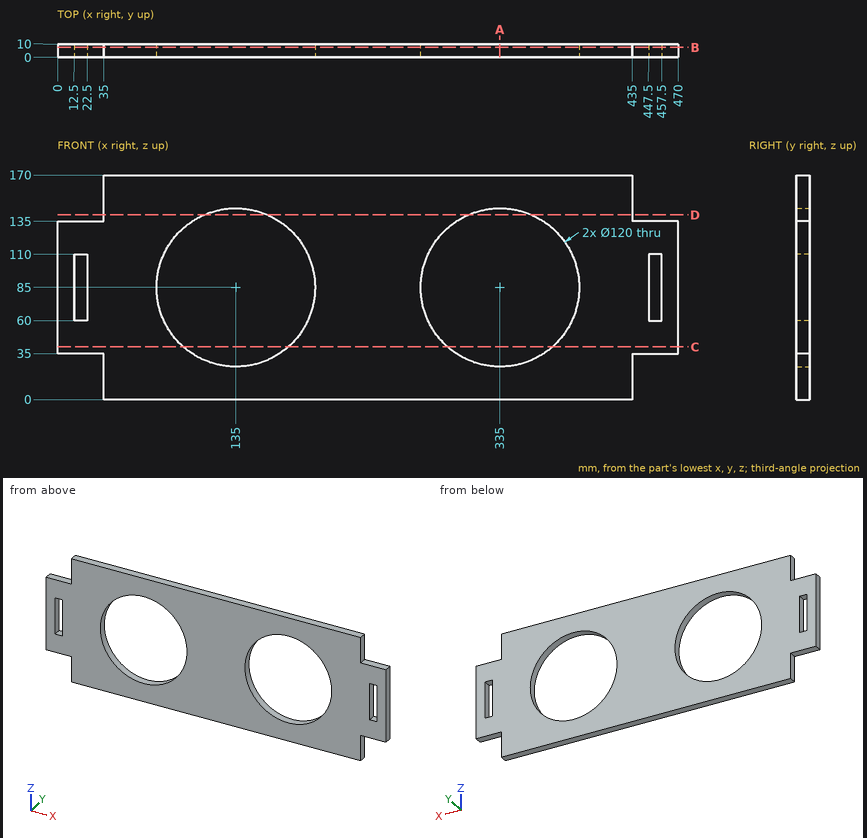
Verification items for this drawing (mm, ordinates from the low corner). Give positions to 0.01 mm unless a question says otherwise; leave off trailing zeros. Order: outer loops, then holes, each group sorted by start corner. A loop starts at its lowest first (then second) coordinate and runs counter-clockwise, first axis right, second up.
1) Cross-section at D-D (z = 140). Record the boundary of the cut face in (x, y), then the cut area to 3 significant figures.
Results are:
outline: (35, 0) - (111.02, 0) - (111.02, 10) - (35, 10) - close; (158.98, 0) - (311.02, 0) - (311.02, 10) - (158.98, 10) - close; (358.98, 0) - (435, 0) - (435, 10) - (358.98, 10) - close
area: 3,040 mm2
2) Gauge pin test, flat ends, axial feed: pin 1 (5 mm diameter, centred on x = 453.5, y = 5.5, fed in from -Z); pin 2 (1.5 mm diameter, centred on y = 2.5, z = 136, fed in from +X); pin 3 (5 mm diameter, centred on x = 18.5, y = 6, fed in from +Z). Record the tip position at first contact, or that the pin passes through.
Results are:
pin 1: stops at z = 35
pin 2: stops at x = 435
pin 3: stops at z = 135
3) Cross-section at B-B (y = 7.5). Record the boundary of the cut face in (x, z), then the cut area to 3 significant figures.
Results are:
outline: (0, 35) - (35, 35) - (35, 0) - (435, 0) - (435, 35) - (470, 35) - (470, 135) - (435, 135) - (435, 170) - (35, 170) - (35, 135) - (0, 135) - close; hole (12.5, 60) - (22.5, 60) - (22.5, 110) - (12.5, 110) - close; hole circle Ø120 at (135, 85); hole circle Ø120 at (335, 85); hole (447.5, 60) - (457.5, 60) - (457.5, 110) - (447.5, 110) - close
area: 51,400 mm2
4) Cross-section at A-A (x = 335). Record the boundary of the cut face in (y, z).
Results are:
outline: (0, 0) - (10, 0) - (10, 25) - (0, 25) - close; (0, 145) - (10, 145) - (10, 170) - (0, 170) - close
5) Material ranges on probe 1 along X at (y, z) = (4, 85); probe 2 along Z at (x, y) = (335, 7.25); probe 3 along X at (y, z) = (3.75, 111), recorded low to high.
Results are:
probe 1: x = 0 to 12.5, 22.5 to 75, 195 to 275, 395 to 447.5, 457.5 to 470
probe 2: z = 0 to 25, 145 to 170
probe 3: x = 0 to 80.93, 189.07 to 280.93, 389.07 to 470
6) Cross-section at C-C (z = 40). Record the boundary of the cut face in (x, y).
Results are:
outline: (0, 0) - (95.31, 0) - (95.31, 10) - (0, 10) - close; (174.69, 0) - (295.31, 0) - (295.31, 10) - (174.69, 10) - close; (374.69, 0) - (470, 0) - (470, 10) - (374.69, 10) - close
